from build123d import *

# Parameters (mm, degrees)
SKETCH1_R               = 6
BOSS_EXTRUDE1_DEPTH     = 10
CHAMFER1_SIZE           = 3.5
CHAMFER1_SIZE2          = 2.020725942
CUT_EXTRUDE1_DEPTH      = 14.114877049
CUT_EXTRUDE1_DEPTH_BACK = 14.114877049
SKETCH2_W               = 12
SKETCH2_H               = 7.979274058
SKETCH3_R               = 2
BOSS_EXTRUDE2_DEPTH     = 19
CHAMFER2_SIZE           = 0.5
FILLET1_R               = 0.25
FILLET2_R               = 1


with BuildPart() as part:
    # Sketch1 → Boss-Extrude1 (new body)
    with BuildSketch(Plane(origin=(0, 0, 0), x_dir=(1, 0, 0), z_dir=(0, 1, 0))):
        with Locations(Location((0, 0, 0), (0, 0, 270))):
            Circle(SKETCH1_R)
    extrude(amount=BOSS_EXTRUDE1_DEPTH)

    # Chamfer1
    chamfer1_edges = [part.edges().sort_by_distance(p)[0] for p in [
        (0, 10, -6),
    ]]
    chamfer1_side = [part.faces().sort_by_distance(p)[0] for p in [
        (0, 10, 0),
    ]]
    chamfer(chamfer1_edges, length=CHAMFER1_SIZE, length2=CHAMFER1_SIZE2, reference=chamfer1_side[0])

    # Sketch2 → Cut-Extrude1 (cut, two sides: drawn at the far end of the back side and taken through both)
    with BuildSketch(Plane.XY.offset(-CUT_EXTRUDE1_DEPTH_BACK)):
        with Locations((0, 3.989637029)):
            Rectangle(SKETCH2_W, SKETCH2_H)
    extrude(amount=CUT_EXTRUDE1_DEPTH + CUT_EXTRUDE1_DEPTH_BACK, mode=Mode.SUBTRACT)

    # Sketch3 → Boss-Extrude2 (add)
    with BuildSketch(Plane(origin=(0, 10, 0), x_dir=(1, 0, 0), z_dir=(0, 1, 0))):
        with Locations(Location((0, 0, 0), (0, 0, 270))):
            Circle(SKETCH3_R)
    extrude(amount=BOSS_EXTRUDE2_DEPTH)

    # Chamfer2
    chamfer2_edges = [part.edges().sort_by_distance(p)[0] for p in [
        (0, 29, -2),
    ]]
    chamfer(chamfer2_edges, length=CHAMFER2_SIZE)

    # Fillet1
    fillet1_edges = [part.edges().sort_by_distance(p)[0] for p in [
        (0, 7.979274058, -6),
    ]]
    fillet(fillet1_edges, radius=FILLET1_R)

    # Fillet2
    fillet2_edges = [part.edges().sort_by_distance(p)[0] for p in [
        (0, 10, -2.5),
    ]]
    fillet(fillet2_edges, radius=FILLET2_R)


solid = part.part
For this review, take the finished solid that the model builds, in its own axes (mm). A direction names the side the tool comes from. Give positions to 0.01 mm unless a question says otherwise; leave off trailing zeros. Loops run counter-clockwise (first coordinate to the right, second up) from the corner with the lowest first, then second, coordinate; pieces in that order, holes last. Notation, with made-up numbers: M 8.5,-5.75 L 21.5,-5.75 A29 ccw 21.5,18.25 Z; hole C 16,22 d5. An arc over 180 degrees is marked long. Put each result on its own line as item: value. Start each with the question number.
(1) Add section A-A, the plane x = 0. Write out the cut boundary in (y, z), then the cut area to 3 significant figures.
(2) Machinability: for faces 1 (the cylindrical face through (-2, 19, 0)), 2 (the flat face through (0, 7.979, 0)), which of the approach directions +Z, -Z, +X, -X, +Y, -Y give a long, thin tool a straight path to every point of the face, cutting with its end or side? Answer none if there is none.
(3) Add section B-B, the plane z = 0. Write out the cut boundary in (x, y).
(4) Wall thickness on L1, parallel to X at y = 15.5, z = 0; L2, parallel to Y at x = 2, z = 0.5; L3, parallel to X at y = 25.25, z = -1.25: over which ranges is each line inside the solid? List them lowest first.
(5) For pin 1 (1.5 mm diameter, centred on y = 17.5, z = 1, fed in from -X); pin 2 (2 mm diameter, centred on x = 2.5, y = 14.5, fed in from +Z); pin 3 (5 mm diameter, centred on x = 1, y = 17, fed in from +Z); pin 4 (3 mm diameter, centred on x = 4, y = 27, fed in from -Z), all flat-tipped, find the tip position at first contact; note any pin that passes through.
(6) Add section C-C, the plane y = 19. Write out the cut boundary in (x, z), then the cut area to 3 significant figures.
Result:
1. outline: M 7.98,-5.07 A0.25 ccw 8.45,-5.19 L 9.87,-2.73 A1 ccw 10,-2.23 L 10,-2 L 28.5,-2 L 29,-1.5 L 29,1.5 L 28.5,2 L 10,2 L 10,2.23 A1 ccw 9.87,2.73 L 8.45,5.19 A0.25 ccw 7.98,5.07 Z
1. area: 92.6 mm^2
2. face 1: +Y
2. face 2: +Z, -Z, +X, -X, -Y
3. outline: M -5.19,8.45 A0.25 ccw -5.07,7.98 L 5.07,7.98 A0.25 ccw 5.19,8.45 L 2.73,9.87 A1 ccw 2.23,10 L 2,10 L 2,28.5 L 1.5,29 L -1.5,29 L -2,28.5 L -2,10 L -2.23,10 A1 ccw -2.73,9.87 Z
4. L1: x = -2 to 2
4. L2: y = 7.98 to 10
4. L3: x = -1.56 to 1.56
5. pin 1: stops at x = -1.98
5. pin 2: stops at z = 1.32
5. pin 3: stops at z = 2
5. pin 4: passes through
6. outline: C 0,0 d4
6. area: 12.6 mm^2
